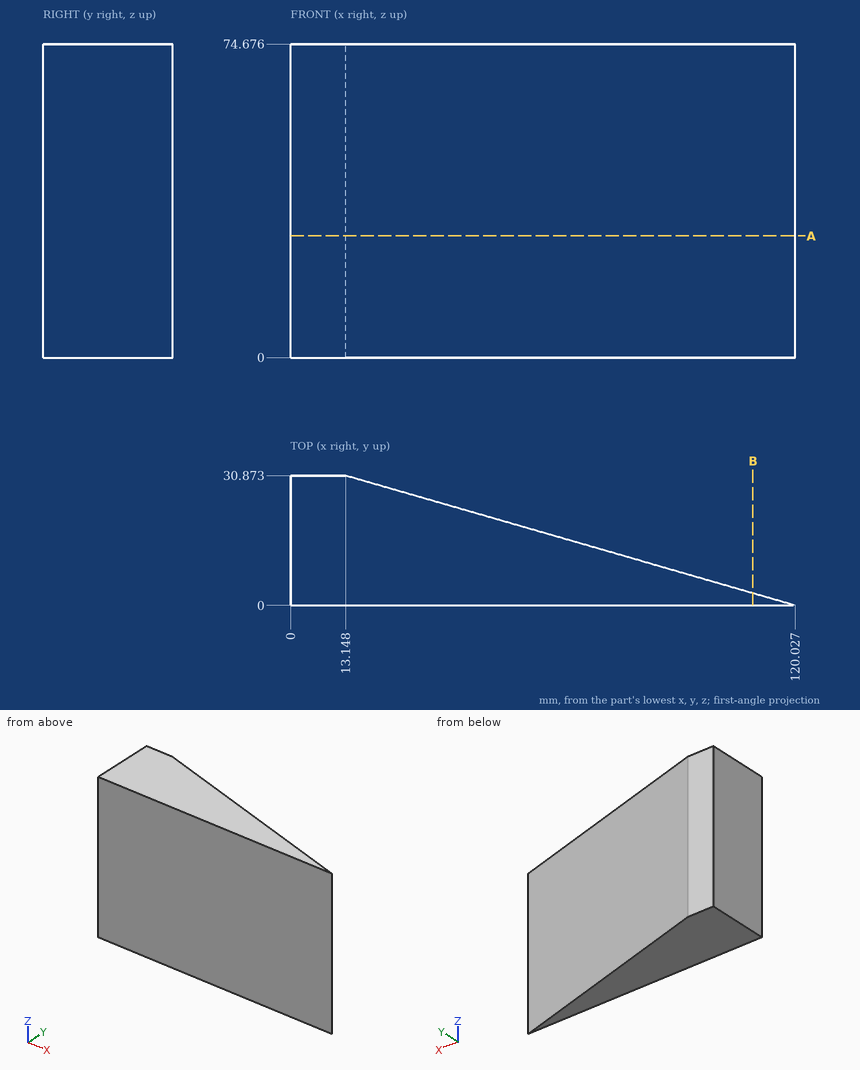
Answer from the drawing. Dimensions are ordinates in mm from the lowest x, y and z of the part. Coordinates: 2 decimals unless noted, no trailing zeros. Order: outer loops, then holes, each group sorted by start corner. A loop starts at its lowest first (then second) coordinate and runs counter-clockwise, first axis right, second up. Notation, with made-up numbers: (-6, 80.5) - (12, 80.5) arc R20 ccw to (12, 101.5) - close; hole circle Ø2 at (-15.75, 42). An arc over 180 degrees is marked (long way). Put each result on its own line as item: value. Start each with the question number.
1) Find the intervals of material crossed by line 1 (Y direction, x = 70.5, z = 44.5) (1 decimal); line 2 (Y direction, x = 107.5, z = 24), in increasing order. Write a range as from..to.
2) Flat-ended cylindrical pins translate along their axes: pin 1 (1 mm diameter, centred on x = 47.5, z = 65, fed in from +Y) (1 decimal); pin 2 (5 mm diameter, centred on x = 31.5, z = 13, fed in from +Y). Find the tip coordinate at first contact, or state that the pin passes through.
3) Find section A-A (z = 29). Give the vertices of the cut face in (x, y), plus the area to 3 significant figures.
4) Find section B-B (x = 110). Give the vertices of the cut face in (y, z).
Results list:
1. line 1: y = 0..14.3
1. line 2: y = 0..3.62
2. pin 1: stops at y = 21.1
2. pin 2: stops at y = 26.29
3. outline: (0, 0) - (120.03, 0) - (13.15, 30.87) - (0, 30.87) - close
3. area: 2,060 mm^2
4. outline: (0, 0) - (2.9, 0) - (2.9, 74.68) - (0, 74.68) - close
